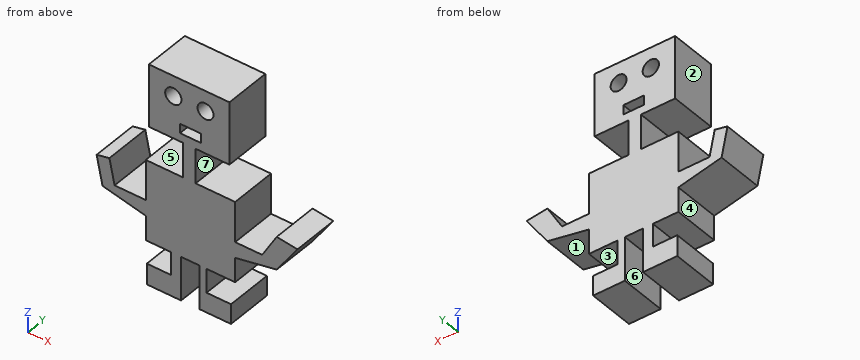
from build123d import *

# Parameters (mm, degrees)
F0_W     = 11.348937
F0_H     = 5.107021
F0_R     = 4.440973
F0_R_2   = 4.340135
F0_W_2   = 6.809362
F0_H_2   = 18.867606
F1_DEPTH = 25.4


with BuildPart() as f1:
    # F0 (on Front) → F1 (new body)
    with BuildSketch(Plane.XZ):
        Polygon((21.988563, 52.914415), (-21.988565, 52.914415), (-21.988565, 18.867606), (-3.262819, 18.867606), (3.546543, 18.867606), (21.988563, 18.867606), align=None)
        with Locations((0.709308, 25.96069)):
            Rectangle(F0_W, F0_H, mode=Mode.SUBTRACT)
        with Locations((-8.653564, 41.849203)):
            Circle(F0_R, mode=Mode.SUBTRACT)
        with Locations((8.937287, 41.849203)):
            Circle(F0_R_2, mode=Mode.SUBTRACT)
        with Locations((0.141862, 9.433803)):
            Rectangle(F0_W_2, F0_H_2)
        Polygon((3.546543, 0), (-3.262819, 0), (-23.690904, 0), (-23.690904, -21.917634), (-23.690904, -30.500267), (-23.690904, -43.835267), (-9.788458, -43.835267), (-4.397713, -43.835267), (5.532607, -43.835267), (9.504734, -43.835267), (25.10952, -43.835267), (25.10952, -30.500267), (25.10952, -21.917634), (25.10952, 0), align=None)
        Polygon((-23.690904, -30.500267), (-23.690904, -21.917634), (-40.714309, -21.917634), (-43.551542, -8.369841), (-50.530179, -9.831335), (-47.290991, -25.298465), align=None)
        Polygon((39.863139, -21.917634), (25.10952, -21.917634), (25.10952, -30.500267), (47.807392, -26.244417), (59.156332, -9.831335), (47.807392, -8.369841), align=None)
        Polygon((-4.397713, -43.835267), (-9.788458, -43.835267), (-9.788458, -56.319095), (-23.123458, -56.319095), (-23.123458, -67.668028), (-4.397713, -67.668028), align=None)
        Polygon((9.504734, -56.886546), (9.504734, -43.835267), (5.532607, -43.835267), (5.532607, -67.668028), (22.839734, -67.668028), (22.839734, -56.886546), align=None)
    extrude(amount=F1_DEPTH)


solid = f1.part
Verification items for the finished model (mm, model axes). Face numbers are marked on the shaded views. A direction names the side the tool comes from. Coordinates: 2 decimals unless noted, no trailing zeros. Order: outer loops, then holes, each group sorted by start corner. A loop starts at its lowest first (then second) coordinate and runs counter-clockwise, first axis right, second up.
1. Sectioned sample at C-C, the plane y = -11.5. Give the number of separate pieces and of enclosed holes in the cut face, and give its area (3 significant figures).
Results found:
separate pieces: 1
enclosed holes: 3
area: 4,640 mm2
2. Go/stop test with flat-tipped pins: pin 1 Ø3 at (y, z) = (-15.5, -51) entering from -X; pin 2 Ø1.5 at (y, z) = (-17.5, -42.5) entering from -X; pin 3 Ø1.5 at (y, z) = (-16.5, 6) entering from +X; pin 4 Ø5 at (x, z) = (-25.5, 35.5) entering from -Y. Record where each tip stops, or that it passes through.
Results found:
pin 1: stops at x = -9.79
pin 2: stops at x = -23.69
pin 3: stops at x = 3.55
pin 4: passes through
3. Sectioned sample at A-A, the plane x = 20. Record the cut outline in (y, z), and give its area (3 significant figures).
Results found:
outline: (-25.4, -67.67) - (0, -67.67) - (0, -56.89) - (-25.4, -56.89) - close; (-25.4, -43.84) - (0, -43.84) - (0, 0) - (-25.4, 0) - close; (-25.4, 18.87) - (0, 18.87) - (0, 52.91) - (-25.4, 52.91) - close
area: 2,250 mm2
4. Sectioned sample at D-D, the plane z = 12.5. Record the cut outline in (x, y).
Results found:
outline: (-3.26, -25.4) - (3.55, -25.4) - (3.55, 0) - (-3.26, 0) - close
5. Release check for a two-part mould opening along Z. For the marked faces 1, 2 and 3 record: +Z half, -Z half, draft (parallel to the pull), parting line (faces both ways), or undercut.
Results found:
face 1: -Z half
face 2: draft
face 3: undercut
6. Set-up check for the marked faces 4, 5, 6 and 7: record each of +Z, -Z, +X, -X, +Y, -Y from which the full face is reachable in a straight line by a thin tool's end or side.
Results found:
face 4: -Z, -X, +Y, -Y
face 5: -X, +Y, -Y
face 6: -Z, +Y, -Y
face 7: +X, +Y, -Y
7. Sectioned sample at B-B, the plane z = -49. Record the cut outline in (x, y), and give its area (3 significant figures).
Results found:
outline: (-9.79, -25.4) - (-4.4, -25.4) - (-4.4, 0) - (-9.79, 0) - close; (5.53, -25.4) - (9.5, -25.4) - (9.5, 0) - (5.53, 0) - close
area: 238 mm2
8. Scan lines: line 1 (Z direction, x = -17, y = -5.25); line 2 (Z direction, x = 17, y = -3.5); line 3 (X direction, y = -5.5, z = 25). Record each from-to range of solid material in increasing order.
Results found:
line 1: z = -67.67 to -56.32, -43.84 to 0, 18.87 to 52.91
line 2: z = -67.67 to -56.89, -43.84 to 0, 18.87 to 52.91
line 3: x = -21.99 to -4.97, 6.38 to 21.99
